Job drawing, mm, ordinate dimensions from the low corner. One solid piece. A direction names the side the tool comes from. Round coordinates to 2 decimals unless told otherwise and drop trailing zeros. Loops run counter-clockwise (first coordinate to the right, second up) from the corner with the lowest first, then second, coordinate; pieces in that order, holes last. Notation, with made-up numbers: M -28,42.5 L 3,42.5 A35 ccw 3,75.5 Z; hole C 39.25,6 d10. An arc over 180 degrees is marked long. One line per item, written item: value.
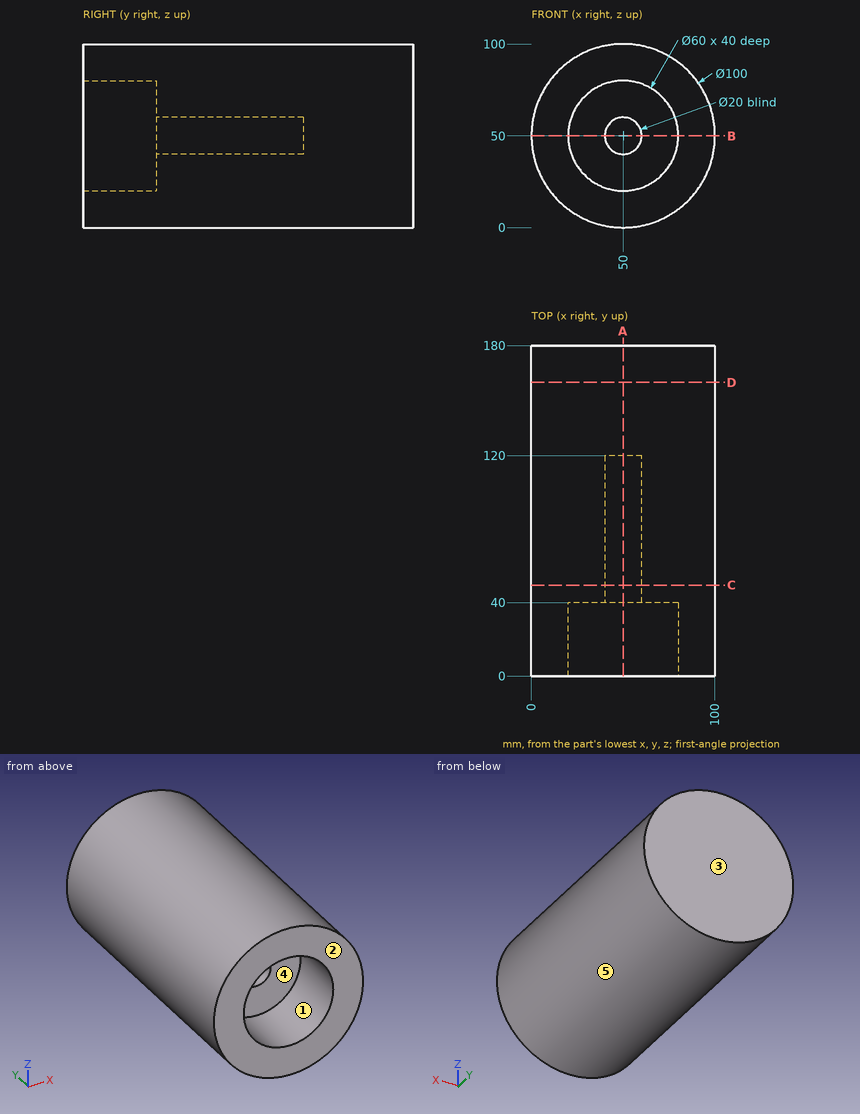
Item 1: Wall check: line 1 along Z through (x, y) = (50, 25); line 2 along Z through (x, y) = (50, 93); line 3 along Y through (x, z) = (39, 35). Give the ranges that are in metal, low to high.
Check values:
line 1: z = 0 to 20, 80 to 100
line 2: z = 0 to 40, 60 to 100
line 3: y = 40 to 180
Item 2: Slice it at D-D, the plane y = 160. Give the cut face in (x, z).
Check values:
outline: C 50,50 d100
Item 3: Slice it at B-B, the plane z = 50. Give the cut face in (x, y), and give its area (3 significant figures).
Check values:
outline: M 0,0 L 20,0 L 20,40 L 40,40 L 40,120 L 60,120 L 60,40 L 80,40 L 80,0 L 100,0 L 100,180 L 0,180 Z
area: 14,000 mm2
Item 4: Slice it at C-C, the plane y = 49.5. Give the cut face in (x, z).
Check values:
outline: C 50,50 d100; hole C 50,50 d20
Item 5: Drop flat-ended pins along their axis: P1, Ø6, axis at x = 53, z = 52, coming from the -Y side; P2, Ø1, axis at y = 138, z = 21.5, coming from the -X side; P3, Ø2, axis at y = 87, z = 68.5, coming from the +X side. Give the stop position or say it passes through.
Check values:
P1: stops at y = 120
P2: stops at x = 8.58
P3: stops at x = 96.84
Item 6: Pull direction Z, two halves, no side cores. Call the marked faces 3, 4 and 5: pulls with the +Z half, pulls with the -Z half, needs draft (parallel to the pull), parting line crosses it, or undercut.
Check values:
face 3: needs draft
face 4: undercut
face 5: parting line crosses it
Item 7: Which spindle directions (+Z, -Z, +X, -X, +Y, -Y) get a long thin tool onto all of the face, cutting with end or side? Do the marked faces 1 and 2. Say none if no direction does.
Check values:
face 1: -Y
face 2: +Z, -Z, +X, -X, -Y
Item 8: Slice it at A-A, the plane x = 50. Give the cut face in (y, z).
Check values:
outline: M 0,0 L 180,0 L 180,100 L 0,100 L 0,80 L 40,80 L 40,60 L 120,60 L 120,40 L 40,40 L 40,20 L 0,20 Z
